Build history of the part. All positions in model axes, mm. A direction names the side the tool comes from. Coordinates: 2 decimals unless noted, no trailing zeros. Loops run counter-clockwise (first coordinate to the right, second up) from the corner with the lowest first, then second, coordinate; pieces in that order, holes last. Notation, with made-up numbers: (6.5, -5) - (59.5, -5) arc R15 cw to (59.5, 19) - close; hole circle Ø7 at (-29.75, -13.5). An arc over 180 degrees is marked (long way). One line per item, written item: value.
```python
from build123d import *

# Parameters (mm, degrees)
IZIM1_R                       = 75
Y_KSEKLIK_EKSTR_ZYON1_DEPTH   = 180
IZIM1_R_2                     = 50
Y_KSEKLIK_EKSTR_ZYON1_2_DEPTH = 180
Y_KSEKLIK_EKSTR_ZYON2_DEPTH   = 20
Y_KSEKLIK_EKSTR_ZYON3_DEPTH   = 20
RADYUS1_R                     = 19
RADYUS1_OF_AYNALAMA1_R        = 19
IZIM4_W                       = 120
IZIM4_H                       = 120
Y_KSEKLIK_EKSTR_ZYON4_DEPTH   = 10
Y_KSEKLIK_EKSTR_ZYON5_REACH   = 597.168
IZIM6_W                       = 100
IZIM6_H                       = 100
RADYUS2_R                     = 20


with BuildPart() as part:
    # izim1 → Y_kseklik-Ekstr_zyon1 (new body)
    with BuildSketch(Plane.XY):
        with Locations(Location((0, 0, 0), (0, 0, 180))):
            Circle(IZIM1_R)
    extrude(amount=Y_KSEKLIK_EKSTR_ZYON1_DEPTH)



with BuildPart() as body_2:
    # izim1 → Y_kseklik-Ekstr_zyon1 2 (new body)
    with BuildSketch(Plane.XY):
        with Locations(Location((0, 500, 0), (0, 0, 180))):
            Circle(IZIM1_R_2)
    extrude(amount=Y_KSEKLIK_EKSTR_ZYON1_2_DEPTH)


with BuildPart() as part_1:
    add(part.part)

    add(body_2.part)  # Y_kseklik-Ekstr_zyon2 merges body 2
    # izim2 → Y_kseklik-Ekstr_zyon2 (add)
    with BuildSketch(Plane.XY):
        with BuildLine():
            Line((50, 500), (98.495702008, 107.476734806))
            ThreePointArc((98.495702008, 107.476734806), (104.263508371, 78.541265575), (114.225589108, 50.769230769))
            ThreePointArc((114.225589108, 50.769230769), (0, -125), (-114.225589108, 50.769230769))
            ThreePointArc((-114.225589108, 50.769230769), (-104.263508371, 78.541265575), (-98.495702008, 107.476734806))
            Line((-98.495702008, 107.476734806), (-50, 500))
            ThreePointArc((-50, 500), (0, 550), (50, 500))
        make_face()
    y_kseklik_ekstr_zyon2 = extrude(amount=-Y_KSEKLIK_EKSTR_ZYON2_DEPTH)

    # izim3 → Y_kseklik-Ekstr_zyon3 (add)
    with BuildSketch(Plane(origin=(0, 0, -20), x_dir=(-1, 0, 0), z_dir=(0, 0, -1))):
        with BuildLine():
            Line((-29.98073719, 498.925105803), (-78.646619041, 105.024408287))
            ThreePointArc((-78.646619041, 105.024408287), (-84.99120604, 73.195392132), (-95.949494851, 42.646153846))
            ThreePointArc((-95.949494851, 42.646153846), (0, -105), (95.949494851, 42.646153846))
            ThreePointArc((95.949494851, 42.646153846), (84.99120604, 73.195392132), (78.646619041, 105.024408287))
            Line((78.646619041, 105.024408287), (29.98073719, 498.925105803))
            ThreePointArc((29.98073719, 498.925105803), (0, 530), (-29.98073719, 498.925105803))
        make_face()
    y_kseklik_ekstr_zyon3 = extrude(amount=Y_KSEKLIK_EKSTR_ZYON3_DEPTH)

    # Radyus1
    radyus1_edges = [part_1.edges().sort_by_distance(p)[0] for p in [
        (0, 530, -20),
        (54.313678116, 301.974757045, -20),
        (84.99120604, 73.195392132, -20),
        (0, -105, -20),
        (-84.99120604, 73.195392132, -20),
        (-54.313678116, 301.974757045, -20),
    ]]
    fillet(radyus1_edges, radius=RADYUS1_R)

    # Aynalama1: Y_kseklik-Ekstr_zyon2, Y_kseklik-Ekstr_zyon3 across plane
    add(y_kseklik_ekstr_zyon2.mirror(Plane.XY.offset(80)))
    add(y_kseklik_ekstr_zyon3.mirror(Plane.XY.offset(80)))

    # Radyus1 of Aynalama1
    radyus1_of_aynalama1_edges = [part_1.edges().sort_by_distance(p)[0] for p in [
        (0, 530, 180),
        (54.313678116, 301.974757045, 180),
        (84.99120604, 73.195392132, 180),
        (0, -105, 180),
        (-84.99120604, 73.195392132, 180),
        (-54.313678116, 301.974757045, 180),
    ]]
    fillet(radyus1_of_aynalama1_edges, radius=RADYUS1_OF_AYNALAMA1_R)

    # izim4 → Y_kseklik-Ekstr_zyon4 (add)
    with BuildSketch(Plane(origin=(0, 0, 160), x_dir=(-1, 0, 0), z_dir=(0, 0, -1))):
        with Locations((0, 270)):
            Rectangle(IZIM4_W, IZIM4_H)
    y_kseklik_ekstr_zyon4 = extrude(amount=Y_KSEKLIK_EKSTR_ZYON4_DEPTH)

    # Aynalama2: Y_kseklik-Ekstr_zyon4 across plane
    add(y_kseklik_ekstr_zyon4.mirror(Plane.XY.offset(80)))

    # izim6 → Y_kseklik-Ekstr_zyon5 (add, up to next)
    with BuildSketch(Plane(origin=(0, 0, 150), x_dir=(-1, 0, 0), z_dir=(0, 0, -1)), mode=Mode.PRIVATE) as y_kseklik_ekstr_zyon5_sk1:
        with Locations((0, 270)):
            Rectangle(IZIM6_W, IZIM6_H)
    y_kseklik_ekstr_zyon5_tool1 = extrude(y_kseklik_ekstr_zyon5_sk1.sketch, amount=Y_KSEKLIK_EKSTR_ZYON5_REACH, mode=Mode.PRIVATE) - part_1.part
    add(y_kseklik_ekstr_zyon5_tool1.solids().sort_by_distance((0, 270, 150))[0])

    # Radyus2
    radyus2_edges = [part_1.edges().sort_by_distance(p)[0] for p in [
        (50, 320, 80),
        (-50, 320, 80),
        (50, 220, 80),
        (-50, 220, 80),
    ]]
    fillet(radyus2_edges, radius=RADYUS2_R)


solid = part_1.part
```
Item 1: Pull direction Z, two halves, no side cores. Call faces 4 (the face through (-59.64, 305.43, -25.42)), 5 (the face through (6.509, 549.575, 81.4)), 6 (the face through (-54.654, 299.217, -39.493)): released by +Z, released by -Z, zero draft, split by the parting line, or undercut.
Check result:
face 4: released by -Z
face 5: undercut
face 6: zero draft
Item 2: Probe probe 1 along Y at (x, z) = (-3.5, 153); probe 2 along Y at (x, z) = (-22, 83.5); probe 3 along Z at (x, y) = (73, 301.5). List the from-to ranges inside material, lowest first. Write a range as from..to.
Check result:
probe 1: y = -74.92..74.92, 210..330, 450.12..549.88
probe 2: y = -71.7..71.7, 220..320, 455.1..544.9
probe 3: z = -20.01..0, 160..180.01
Item 3: Cut at B-B, the plane x = 0. Give the number of separate pieces and of enclosed holes in the cut face, then the cut area to 3 significant figures.
Check result:
separate pieces: 1
enclosed holes: 2
area: 109,000 mm^2
Item 4: Drop flat-ended pins along their axis: P1, Ø18, axis at x = -11.5, z = 51, coming from the -Y side; P2, Ø3, axis at y = 298, z = 136, coming from the +X side; P3, Ø3, axis at x = 15.5, z = 5.5, coming from the -Y side. Give the stop position or say it passes through.
Check result:
P1: stops at y = -74.96
P2: stops at x = 50
P3: stops at y = -73.68
Item 5: Cut at A-A, the plane z = 126. Write the cut outline in (x, y), then the cut area to 3 significant figures.
Check result:
outline: circle Ø150 at (0, 0); (-50, 240) arc R20 ccw to (-30, 220) - (30, 220) arc R20 ccw to (50, 240) - (50, 300) arc R20 ccw to (30, 320) - (-30, 320) arc R20 ccw to (-50, 300) - close; circle Ø100 at (0, 500)
area: 35,200 mm^2
Item 6: Tool access for faces 1 (the face through (50, 270, 81)), 2 (the face through (43.986, 314.297, 79.02)), 3 (the face through (2, 122, 160)): list every direction of +Z, -Z, +X, -X, +Y, -Y with a clear straight run to the whole face (end or side of a thin tool).
Check result:
face 1: +X, +Y
face 2: +X
face 3: none
